```python
from build123d import *

# Parameters (mm, degrees)
BOSS_EXTRUDE1_DEPTH         = 28
SHELL1_T                    = -2
CUT_EXTRUDE1_START          = -10
SKETCH2_R                   = 2
CUT_EXTRUDE1_DEPTH          = 10
M3_TAPPED_HOLE1_D           = 2.5
M3_TAPPED_HOLE1_DEPTH       = 2
M3_TAPPED_HOLE1_CSINK_D     = 3.5
M3_TAPPED_HOLE1_CSINK_ANGLE = 90
M3_TAPPED_HOLE2_D           = 2.5
M3_TAPPED_HOLE2_CSINK_D     = 3.5
M3_TAPPED_HOLE2_CSINK_ANGLE = 90


with BuildPart() as part:
    # Sketch1 → Boss-Extrude1 (new body)
    with BuildSketch(Plane.XY):
        with BuildLine():
            Line((-48.5, 63.875), (48.5, 63.875))
            ThreePointArc((48.5, 63.875), (51.328427125, 62.703427125), (52.5, 59.875))
            Line((52.5, 59.875), (52.5, -86.875))
            ThreePointArc((52.5, -86.875), (51.328427125, -89.703427125), (48.5, -90.875))
            Line((48.5, -90.875), (-48.5, -90.875))
            ThreePointArc((-48.5, -90.875), (-51.328427125, -89.703427125), (-52.5, -86.875))
            Line((-52.5, -86.875), (-52.5, 59.875))
            ThreePointArc((-52.5, 59.875), (-51.328427125, 62.703427125), (-48.5, 63.875))
        make_face()
    extrude(amount=-BOSS_EXTRUDE1_DEPTH)

    # Shell1
    shell1_openings = [part.faces().sort_by_distance(p)[0] for p in [
        (0, -13.5, 0),
    ]]
    offset(amount=SHELL1_T, openings=shell1_openings, kind=Kind.INTERSECTION)

    # Sketch2 → Cut-Extrude1 (cut)
    with BuildSketch(Plane(origin=(0, 0, -28), x_dir=(-1, 0, 0), z_dir=(0, 0, -1)).offset(CUT_EXTRUDE1_START)):
        with Locations((-37.5, 48.875)):
            Circle(SKETCH2_R)
        with Locations((37.5, 48.875)):
            Circle(SKETCH2_R)
        with Locations((37.5, -36.125)):
            Circle(SKETCH2_R)
        with Locations((-37.5, -36.125)):
            Circle(SKETCH2_R)
        with BuildLine():
            Line((-50.5, -50.875), (50.5, -50.875))
            Line((50.5, -50.875), (50.5, -86.875))
            ThreePointArc((50.5, -86.875), (49.914213562, -88.289213562), (48.5, -88.875))
            Line((48.5, -88.875), (-48.5, -88.875))
            ThreePointArc((-48.5, -88.875), (-49.914213562, -88.289213562), (-50.5, -86.875))
            Line((-50.5, -86.875), (-50.5, -50.875))
        make_face()
    extrude(amount=CUT_EXTRUDE1_DEPTH, mode=Mode.SUBTRACT)

    # M3 Tapped Hole1
    with Locations(Plane(origin=(52.5, 0, 0), x_dir=(0, 0, -1), z_dir=(1, 0, 0))):
        with Locations((8, 0)):
            CounterSinkHole(M3_TAPPED_HOLE1_D / 2, M3_TAPPED_HOLE1_CSINK_D / 2, depth=M3_TAPPED_HOLE1_DEPTH, counter_sink_angle=M3_TAPPED_HOLE1_CSINK_ANGLE)

    # M3 Tapped Hole2 (through all)
    with Locations(Plane.ZY.offset(52.5)):
        with Locations((-8, 0)):
            CounterSinkHole(M3_TAPPED_HOLE2_D / 2, M3_TAPPED_HOLE2_CSINK_D / 2, counter_sink_angle=M3_TAPPED_HOLE2_CSINK_ANGLE)


solid = part.part
```
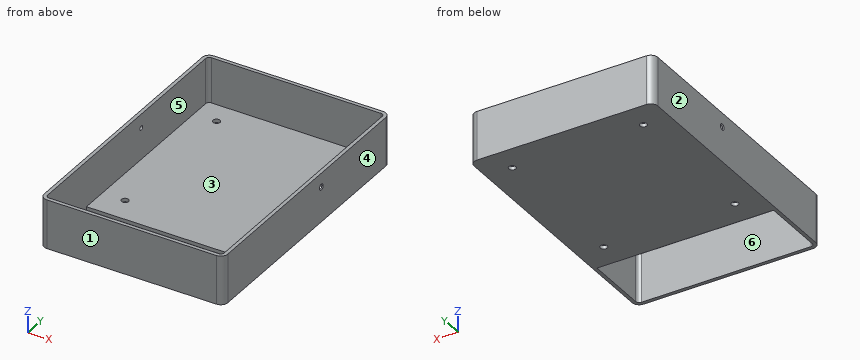
For this review, take the finished solid that the model builds, in its own axes (mm). Face numbers are marked on the shaded views. A direction names the side the tool comes from. Give positions to 0.01 mm unless a question says otherwise; leave off trailing zeros. Write each loop counter-clockwise with the first axis right and the second up, starting at its lowest first coordinate (ties: lowest second). Pieces come first, ordered by that corner, then holes.
Item 1: Take a section at C-C (y = -47). Give the boundary of the cut face in (x, z), and give its area (3 significant figures).
Item 2: Take a section at B-B (x = -44.5). Give the boundary of the cut face in (y, z) (3 decimals).
Item 3: Take a section at A-A (x = 37.5). Give the boundary of the cut face in (y, z) (3 decimals), and give its area (4 significant figures).
Item 4: Wall thickness on probe 1 along Y at (x, z) = (-37.5, -26.55) (3 decimals); probe 2 along Y at (x, z) = (-4.5, -21.5) (3 decimals); probe 3 along X at (y, z) = (14.5, -20): over which ranges is each line inside the solid? List them lowest first.
Item 5: The part is to be moulded in two halves that separate along Y. For the marked faces 1, 2 and 3, say which applies: +Y half, -Y half, draft (parallel to the pull), parting line (faces both ways), or undercut.
Item 6: Machinability: for the marked faces 4, 5 and 6, which of the approach directions +Z, -Z, +X, -X, +Y, -Y give a long, thin tool a straight path to every point of the face, cutting with its end or side? Answer none if there is none.
Item 7: Take a section at D-D (z = -3.5). Give the boundary of the cut face in (x, y) (3 decimals).
Item 8: Insertion check: P1, Ø6.5, axis at x = 37.5, y = 48.875, coming from the +Z side; P2, Ø3, axis at y = 0, z = -8, coming from the +X side. Each pin has a flat end and moves straight along its axis. Give the tip position at first contact, or say it passes through.
Established:
1. outline: (-52.5, -28) - (52.5, -28) - (52.5, 0) - (50.5, 0) - (50.5, -26) - (-50.5, -26) - (-50.5, 0) - (-52.5, 0) - close
1. area: 314 mm2
2. outline: (-90.875, -28) - (-88.875, -28) - (-88.875, 0) - (-90.875, 0) - close; (-50.875, -28) - (63.875, -28) - (63.875, 0) - (61.875, 0) - (61.875, -26) - (-50.875, -26) - close
3. outline: (-90.875, -28) - (-88.875, -28) - (-88.875, 0) - (-90.875, 0) - close; (-50.875, -28) - (-38.125, -28) - (-38.125, -26) - (-50.875, -26) - close; (-34.125, -28) - (46.875, -28) - (46.875, -26) - (-34.125, -26) - close; (50.875, -28) - (63.875, -28) - (63.875, 0) - (61.875, 0) - (61.875, -26) - (50.875, -26) - close
3. area: 321.5 mm2
4. probe 1: y = -90.875 to -88.875, -50.875 to -38.125, -34.125 to 46.875, 50.875 to 63.875
4. probe 2: y = -90.875 to -88.875, 61.875 to 63.875
4. probe 3: x = -52.5 to -50.5, 50.5 to 52.5
5. face 1: -Y half
5. face 2: draft
5. face 3: undercut
6. face 4: +Z, -Z, +X, +Y, -Y
6. face 5: +Z
6. face 6: +Z, -Z
7. outline: (-52.5, -86.875) arc R4 ccw to (-48.5, -90.875) - (48.5, -90.875) arc R4 ccw to (52.5, -86.875) - (52.5, 59.875) arc R4 ccw to (48.5, 63.875) - (-48.5, 63.875) arc R4 ccw to (-52.5, 59.875) - close; hole (-50.5, -86.875) arc R2 ccw to (-48.5, -88.875) - (48.5, -88.875) arc R2 ccw to (50.5, -86.875) - (50.5, 59.875) arc R2 ccw to (48.5, 61.875) - (-48.5, 61.875) arc R2 ccw to (-50.5, 59.875) - close
8. P1: stops at z = -26
8. P2: stops at x = 52.25
